Geometry check sheet. Reference: the model listing, model coordinates, mm. Round coordinates to 2 decimals unless told otherwise and drop trailing zeros. Write each loop counter-clockwise with the first axis right and the second up, starting at its lowest first coordinate (ties: lowest second). Pieces come first, ordered by that corner, then holes. Notation, with made-up numbers: (62, 22.25) - (93, 22.25) arc R16 ccw to (93, 31.25) - close; hole circle Ø9 at (-25.5, 71). An arc over 180 degrees is marked (long way). Return JSON: item names as keys, results as strings. Group by question number.
from build123d import *

# Parameters (mm, degrees)
BOSS_EXTRUDE1_DEPTH = 4
FILLET1_R           = 40
SKETCH2_R           = 3
CUT_EXTRUDE1_DEPTH  = 4
SKETCH3_R           = 2
SKETCH3_R_2         = 2.5
CUT_EXTRUDE2_DEPTH  = 4
FILLET2_R           = 80
FILLET3_R           = 50


with BuildPart() as part:
    # Sketch1 → Boss-Extrude1 (new body)
    with BuildSketch(Plane(origin=(0, 0, 0), x_dir=(1, 0, 0), z_dir=(0, 1, 0))):
        Polygon((-100, 100), (100, 100), (100, -100), (-100, -100), (-100, -50), (-200, -50), (-200, 50), (-100, 50), align=None)
    extrude(amount=BOSS_EXTRUDE1_DEPTH)

    # Fillet1
    fillet1_edges = [part.edges().sort_by_distance(p)[0] for p in [
        (-100, 2, 50),
        (-200, 2, 50),
        (-200, 2, -50),
        (-100, 2, -50),
    ]]
    fillet(fillet1_edges, radius=FILLET1_R)

    # Sketch2 → Cut-Extrude1 (cut)
    with BuildSketch(Plane(origin=(0, 4, 0), x_dir=(1, 0, 0), z_dir=(0, 1, 0))):
        with Locations(Location((42.425, 42.425, 0), (0, 0, 270))):
            Circle(SKETCH2_R)
        with Locations(Location((42.425, -42.425, 0), (0, 0, 270))):
            Circle(SKETCH2_R)
        with Locations(Location((-42.425, -42.425, 0), (0, 0, 270))):
            Circle(SKETCH2_R)
        with Locations(Location((-42.425, 42.425, 0), (0, 0, 270))):
            Circle(SKETCH2_R)
    extrude(amount=-CUT_EXTRUDE1_DEPTH, mode=Mode.SUBTRACT)

    # Sketch3 → Cut-Extrude2 (cut)
    with BuildSketch(Plane(origin=(0, 4, 0), x_dir=(1, 0, 0), z_dir=(0, 1, 0))):
        with Locations(Location((-114.5, -25.5, 0), (0, 0, 270))):
            Circle(SKETCH3_R)
        with Locations(Location((-106.5, 23.5, 0), (0, 0, 270))):
            Circle(SKETCH3_R_2)
        with Locations(Location((-153.5, 23.5, 0), (0, 0, 270))):
            Circle(SKETCH3_R_2)
        with Locations(Location((-153.5, -23.5, 0), (0, 0, 270))):
            Circle(SKETCH3_R_2)
        with Locations(Location((-106.5, -23.5, 0), (0, 0, 270))):
            Circle(SKETCH3_R_2)
        with Locations(Location((-145.5, -25.5, 0), (0, 0, 270))):
            Circle(SKETCH3_R)
        with Locations(Location((-145.5, 25.5, 0), (0, 0, 270))):
            Circle(SKETCH3_R)
        with Locations(Location((-114.5, 25.5, 0), (0, 0, 270))):
            Circle(SKETCH3_R)
    extrude(amount=-CUT_EXTRUDE2_DEPTH, mode=Mode.SUBTRACT)

    # Fillet2
    fillet2_edges = [part.edges().sort_by_distance(p)[0] for p in [
        (100, 2, 100),
        (100, 2, -100),
    ]]
    fillet(fillet2_edges, radius=FILLET2_R)

    # Fillet3
    fillet3_edges = [part.edges().sort_by_distance(p)[0] for p in [
        (-100, 2, -100),
        (-100, 2, 100),
    ]]
    fillet(fillet3_edges, radius=FILLET3_R)


solid = part.part
1. Depth check by flat-ended pin: pin 1 Ø1.5 at (y, z) = (0.5, -36) entering from +X; pin 2 Ø4.5 at (x, z) = (-114.5, -25.5) entering from -Y; pin 3 Ø1.2 at (x, y) = (-148.5, 1.5) entering from +Z; pin 4 Ø5 at (x, z) = (42.425, 42.425) entering from -Y. Enter the tip coordinate at first touch or a pass-through.
2. Section check C-C (x = 49). Enter the section's corners in (y, z), and give its area (3 significant figures).
3. Mould release check, pull along Z, two halves, no side actions. Record for faces 1 (the face through (-48, 4, -1)), 2 (the face through (-119.183, 2.028, -55.844)), 3 (the face through (42.56, 2.03, -45.42)), 4 (the face through (-118.655, 2.028, 56.171)): pulls with the +Z half, pulls with the -Z half, needs draft (parallel to the pull), parting line crosses it, or undercut.
4. Section check B-B (z = 55.5). Enter the section's corners in (x, y).
5. Section check A-A (y = 1.6). State how many separate pieces and enclosed holes the cut face has, and give its area (3 significant figures).
6. Material ranges on line 1 along X through (y, z) = (3.5, 23); line 2 along X through (y, z) = (1.55, 41); line 3 along Z through (x, y) = (42.5, 1.1), recorded low to high.
Result sheet:
{
 "1": {"pin 1": "stops at x = 98.53", "pin 2": "stops at y = 0", "pin 3": "stops at z = 50", "pin 4": "passes through"},
 "2": {"outline": "(0, -94.56) - (4, -94.56) - (4, 94.56) - (0, 94.56) - close", "area": "756 mm²"},
 "3": {"face 1": "needs draft", "face 2": "pulls with the -Z half", "face 3": "undercut", "face 4": "pulls with the +Z half"},
 "4": {"outline": "(-119.76, 0) - (91.69, 0) - (91.69, 4) - (-119.76, 4) - close"},
 "5": {"separate pieces": "1", "enclosed holes": "12", "area": "46,500 mm²"},
 "6": {"line 1": "x = -197.83 to -155.95, -151.05 to -108.95, -104.05 to 99.94", "line 2": "x = -185.28 to -45.06, -39.79 to 39.79, 45.06 to 97.19", "line 3": "z = -96.77 to -45.42, -39.43 to 39.43, 45.42 to 96.77"}
}
